from build123d import *

# Parameters (mm, degrees)
SKETCH_2_W                            = 2.5
SKETCH_2_H                            = 8
CUT_EXTRUDE_1_DEPTH                   = 10
SKETCH_5_R                            = 1.5
CUT_EXTRUDE_4_DEPTH                   = 0.15
SKETCH_7_R                            = 0.5
EXTRUDE_1_DEPTH                       = 0.4
DOME_1_FACE_RADIUS                    = 0.5
DOME_1_HEIGHT                         = 0.25
PATTERN_CIRCULAR_1_COUNT              = 2
PATTERN_CIRCULAR_1_COPY_1_FACE_RADIUS = 0.5
PATTERN_CIRCULAR_1_COPY_1_HEIGHT      = 0.25


with BuildPart() as part:
    # Эскиз1 → Повернуть1 (revolve)
    with BuildSketch(Plane(origin=(0, 0, 0), x_dir=(0, 0, -1), z_dir=(1, 0, 0))):
        with BuildLine():
            Line((4.7, 20), (4.7, 16))
            ThreePointArc((4.7, 16), (4.57524704, 14.75), (4.7, 13.5))
            Line((4.7, 13.5), (4.7, 9))
            Line((4.7, 9), (7, 9))
            Line((7, 9), (7, 8))
            Line((7, 8), (6, 8))
            Line((6, 8), (6, 1.4))
            ThreePointArc((6, 1.4), (5.882842712, 1.117157288), (5.6, 1))
            Line((5.6, 1), (5.2, 1))
            ThreePointArc((5.2, 1), (4.917157288, 0.882842712), (4.8, 0.6))
            Line((4.8, 0.6), (4.8, 0.4))
            ThreePointArc((4.8, 0.4), (4.682842712, 0.117157288), (4.4, 0))
            Line((4.4, 0), (3, 0))
            Line((3, 0), (3, 8))
            Line((3, 8), (4, 8))
            Line((4, 8), (4.4, 20))
            Line((4.4, 20), (4.7, 20))
        make_face()
    revolve(axis=Axis((0, 0, 0), (0, 1, 0)))

    # Эскиз2 → Вырез-Вытянуть1 (cut, symmetric)
    with BuildSketch(Plane.XY):
        with Locations((-5.75, 4)):
            Rectangle(SKETCH_2_W, SKETCH_2_H)
        with Locations((5.75, 4)):
            Rectangle(SKETCH_2_W, SKETCH_2_H)
    extrude(amount=CUT_EXTRUDE_1_DEPTH, both=True, mode=Mode.SUBTRACT)

    # Эскиз5 → Вырез-Вытянуть4 (cut)
    with BuildSketch(Plane.XY.offset(4.7)):
        with Locations((0, 14.75)):
            Circle(SKETCH_5_R)
    cut_extrude_4 = extrude(amount=-CUT_EXTRUDE_4_DEPTH, mode=Mode.SUBTRACT)

    # Эскиз7 → Бобышка-Вытянуть1 (add)
    with BuildSketch(Plane.XY.offset(4.55)):
        with Locations(Location((0, 14.75, 0), (0, 0, 192.319298658))):
            Circle(SKETCH_7_R)
    extrude_1 = extrude(amount=EXTRUDE_1_DEPTH)

    # Купол1: a dome of height H over a round flat face of radius A is a cap of a sphere of radius (A * A + H * H) / (2 * H)
    dome_1_r = (DOME_1_FACE_RADIUS * DOME_1_FACE_RADIUS + DOME_1_HEIGHT * DOME_1_HEIGHT) / (2 * DOME_1_HEIGHT)
    dome_1_base = Plane((0, 14.75, 4.95), z_dir=(0, 0, 1))
    with Locations(dome_1_base.offset(DOME_1_HEIGHT - dome_1_r)):
        dome_1_ball = Sphere(dome_1_r, mode=Mode.PRIVATE)
    add(split(dome_1_ball, bisect_by=dome_1_base, keep=Keep.TOP, mode=Mode.PRIVATE))

    # Круговой массив1: Вырез-Вытянуть4, Бобышка-Вытянуть1 ×2 about axis
    pattern_circular_1_axis = Axis((0, 9, 0), (0, -1, 0))
    add([cut_extrude_4.rotate(pattern_circular_1_axis, i * 360 / PATTERN_CIRCULAR_1_COUNT) for i in range(1, PATTERN_CIRCULAR_1_COUNT)], mode=Mode.SUBTRACT)
    add([extrude_1.rotate(pattern_circular_1_axis, i * 360 / PATTERN_CIRCULAR_1_COUNT) for i in range(1, PATTERN_CIRCULAR_1_COUNT)])

    # Круговой массив1 copy 1: a dome of height H over a round flat face of radius A is a cap of a sphere of radius (A * A + H * H) / (2 * H)
    pattern_circular_1_copy_1_r = (PATTERN_CIRCULAR_1_COPY_1_FACE_RADIUS * PATTERN_CIRCULAR_1_COPY_1_FACE_RADIUS + PATTERN_CIRCULAR_1_COPY_1_HEIGHT * PATTERN_CIRCULAR_1_COPY_1_HEIGHT) / (2 * PATTERN_CIRCULAR_1_COPY_1_HEIGHT)
    pattern_circular_1_copy_1_base = Plane((0, 14.75, -4.95), z_dir=(0, 0, -1))
    with Locations(pattern_circular_1_copy_1_base.offset(PATTERN_CIRCULAR_1_COPY_1_HEIGHT - pattern_circular_1_copy_1_r)):
        pattern_circular_1_copy_1_ball = Sphere(pattern_circular_1_copy_1_r, mode=Mode.PRIVATE)
    add(split(pattern_circular_1_copy_1_ball, bisect_by=pattern_circular_1_copy_1_base, keep=Keep.TOP, mode=Mode.PRIVATE))


solid = part.part
Could you check a few things on this model? Use its own coordinates, in mm. A direction names the side the tool comes from. Round coordinates to 2 decimals unless told otherwise and drop trailing zeros. Order: outer loops, then holes, each group sorted by start corner. A loop starts at its lowest first (then second) coordinate and runs counter-clockwise, first axis right, second up.
(1) Imagine slicing it at D-D (x = -5.25). Write out the boundary of the cut face in (y, z).
Response values:
outline: (8, -4.63) - (9, -4.63) - (9, 4.63) - (8, 4.63) - close
(2) Imagine slicing it at A-A (z = 0). Write out the boundary of the cut face in (x, y).
Response values:
outline: (-7, 8) - (-4.5, 8) - (-4.5, 0.01) arc R0.4 ccw to (-4.4, 0) - (-3, 0) - (-3, 8) - (-4, 8) - (-4.4, 20) - (-4.7, 20) - (-4.7, 16) arc R6.32 cw to (-4.7, 13.5) - (-4.7, 9) - (-7, 9) - close; (3, 0) - (4.4, 0) arc R0.4 ccw to (4.5, 0.01) - (4.5, 8) - (7, 8) - (7, 9) - (4.7, 9) - (4.7, 13.5) arc R6.32 cw to (4.7, 16) - (4.7, 20) - (4.4, 20) - (4, 8) - (3, 8) - close
(3) Which directions (+Z, -Z, +X, -X, +Y, -Y) give clear straight access to the entire face, cutting with the end or side of a thin tool? Please do faces 4 (the cylindrical face through (1.8, 17.97, -4.34)), 5 (the cylindrical face through (0, 15.25, -4.75)), 6 (the flat face through (-4.5, 4, 0)), 7 (the flat face through (0, 14, 4.55)), 8 (the cylindrical face through (0, 5, -6)).
Response values:
face 4: +Y
face 5: -Z
face 6: +Z, -Z, -X, -Y
face 7: +Z
face 8: -Z, -Y
(4) I'm going to push flat-ended pins straight in: pin 1 (1.1 mm diameter, centred on x = 0, y = 13.5, fed in from -Z); pin 2 (2.5 mm diameter, centred on x = -2, z = 0.5, fed in from +Y); pin 3 (1.5 mm diameter, centred on x = -5.5, z = -1, fed in from -Y); pin 4 (1 mm diameter, centred on x = -4.5, z = -1, fed in from -Y). Where does each tip first touch, or does it pass through?
Response values:
pin 1: stops at z = -4.7
pin 2: stops at y = 8
pin 3: stops at y = 8
pin 4: stops at y = 0
(5) If we mould it in two halves opening along Z, with no side actions, what happens to faces 1 (the conical face through (-1.26, 14.08, -4.01)), 2 (the flat face through (4.5, 4, 0)), 3 (the flat face through (0, 14, -4.55))? For each: released by +Z, released by -Z, zero draft, split by the parting line, or undercut.
Response values:
face 1: undercut
face 2: zero draft
face 3: released by -Z
(6) Imagine slicing it at B-B (y = 5.5). Write out the boundary of the cut face in (x, z).
Response values:
outline: (-4.5, -3.97) arc R6 ccw to (4.5, -3.97) - (4.5, 3.97) arc R6 ccw to (-4.5, 3.97) - close; hole circle Ø6 at (0, 0)
(7) Imagine slicing it at C-C (x = 5.75). Write out the boundary of the cut face in (y, z), plus the area to 3 significant figures.
Response values:
outline: (8, -3.99) - (9, -3.99) - (9, 3.99) - (8, 3.99) - close
area: 7.98 mm2
(8) Please list where these lines run through material, in increasing order: line 1 along Z through (x, y) = (0, 2.5); line 2 along X through (y, z) = (3, 0); line 3 along Y through (x, z) = (-4, 5.5).
Response values:
line 1: z = -6 to -3, 3 to 6
line 2: x = -4.5 to -3, 3 to 4.5
line 3: y = 8 to 9
